Check sheet for the modelled part. Datum: model origin and axes. Units: mm. Face numbers are marked on the shaded views. A direction names the side the tool comes from. Round coordinates to 2 decimals unless told otherwise and drop trailing zeros. Order: outer loops, then holes, each group sorted by start corner. A loop starts at its lowest first (then second) coordinate and runs counter-clockwise, first axis right, second up. Notation, with made-up numbers: (36, -17.75) -> (50, -17.75) arc R10 cw to (50, -3.75) -> close; hole circle Ø10 at (11, -6.75). An arc over 180 degrees is marked (long way). Answer in a Markdown table with one row per item.
from build123d import *
from build123d.topology import SkipClean

# Parameters (mm, degrees)
SKETCH1_R           = 2
SKETCH1_R_2         = 2.5
BOSS_EXTRUDE1_DEPTH = 5
SKETCH2_R           = 3
CUT_EXTRUDE2_DEPTH  = 5
SKETCH6_R           = 40
SKETCH6_R_2         = 38
BOSS_EXTRUDE2_DEPTH = 10
CUT_EXTRUDE3_DEPTH  = 29
FILLET1_R           = 5


with BuildPart() as part:
    # Sketch1 → Boss-Extrude1 (new, symmetric)
    with SkipClean():  # the faces are left unmerged after this step: merging them gives an invalid solid
        with BuildSketch(Plane.XY):
            with BuildLine():
                Line((0, 40), (130, 40))
                ThreePointArc((130, 40), (170, 0), (130, -40))
                Line((130, -40), (0, -40))
                ThreePointArc((0, -40), (-40, 0), (0, 40))
            make_face()
            with Locations((0, 34)):
                Circle(SKETCH1_R, mode=Mode.SUBTRACT)
            with Locations((29.444863729, 17)):
                Circle(SKETCH1_R, mode=Mode.SUBTRACT)
            with Locations((29.444863729, -17)):
                Circle(SKETCH1_R, mode=Mode.SUBTRACT)
            with Locations((0, -34)):
                Circle(SKETCH1_R, mode=Mode.SUBTRACT)
            with Locations((-29.444863729, -17)):
                Circle(SKETCH1_R, mode=Mode.SUBTRACT)
            with Locations((-29.444863729, 17)):
                Circle(SKETCH1_R, mode=Mode.SUBTRACT)
            with Locations(Location((130, -34, 0), (0, 0, 180))):
                Circle(SKETCH1_R, mode=Mode.SUBTRACT)
            with Locations(Location((159.444863729, 17, 0), (0, 0, 180))):
                Circle(SKETCH1_R, mode=Mode.SUBTRACT)
            with Locations(Location((159.444863729, -17, 0), (0, 0, 180))):
                Circle(SKETCH1_R, mode=Mode.SUBTRACT)
            with Locations(Location((100.555136271, -17, 0), (0, 0, 180))):
                Circle(SKETCH1_R, mode=Mode.SUBTRACT)
            with Locations(Location((100.555136271, 17, 0), (0, 0, 180))):
                Circle(SKETCH1_R, mode=Mode.SUBTRACT)
            with Locations(Location((130, 34, 0), (0, 0, 180))):
                Circle(SKETCH1_R, mode=Mode.SUBTRACT)
            with Locations((55, 30)):
                Circle(SKETCH1_R_2, mode=Mode.SUBTRACT)
            with Locations(Location((75, 30, 0), (0, 0, 180))):
                Circle(SKETCH1_R_2, mode=Mode.SUBTRACT)
            with Locations((75, -30)):
                Circle(SKETCH1_R_2, mode=Mode.SUBTRACT)
            with Locations(Location((55, -30, 0), (0, 0, 180))):
                Circle(SKETCH1_R_2, mode=Mode.SUBTRACT)
            with BuildLine():
                ThreePointArc((25, 0), (0, 25), (-25, 0))
                ThreePointArc((-25, 0), (0, -25), (25, 0))
            make_face(mode=Mode.SUBTRACT)
            with BuildLine():
                ThreePointArc((155, 0), (130, -25), (105, 0))
                ThreePointArc((105, 0), (130, 25), (155, 0))
            make_face(mode=Mode.SUBTRACT)
        extrude(amount=BOSS_EXTRUDE1_DEPTH, both=True)
    add(part.part.scale(1), mode=Mode.REPLACE)  # the faces are merged on a copy

    # Sketch2 → Cut-Extrude2 (cut)
    with BuildSketch(Plane(origin=(0, 0, -5), x_dir=(-1, 0, 0), z_dir=(0, 0, -1))):
        with Locations((-130, 34)):
            Circle(SKETCH2_R)
        with Locations((-100.555136271, 17)):
            Circle(SKETCH2_R)
        with Locations((-100.555136271, -17)):
            Circle(SKETCH2_R)
        with Locations((-130, -34)):
            Circle(SKETCH2_R)
        with Locations((-159.444863729, -17)):
            Circle(SKETCH2_R)
        with Locations((-159.444863729, 17)):
            Circle(SKETCH2_R)
        with Locations(Location((29.444863729, 17, 0), (0, 0, 180))):
            Circle(SKETCH2_R)
        with Locations(Location((29.444863729, -17, 0), (0, 0, 180))):
            Circle(SKETCH2_R)
        with Locations(Location((0, -34, 0), (0, 0, 180))):
            Circle(SKETCH2_R)
        with Locations(Location((-29.444863729, -17, 0), (0, 0, 180))):
            Circle(SKETCH2_R)
        with Locations(Location((-29.444863729, 17, 0), (0, 0, 180))):
            Circle(SKETCH2_R)
        with Locations(Location((0, 34, 0), (0, 0, 180))):
            Circle(SKETCH2_R)
    extrude(amount=-CUT_EXTRUDE2_DEPTH, mode=Mode.SUBTRACT)

    # Sketch6 → Boss-Extrude2 (add)
    # profile 1 of 2: a face of its own
    with SkipClean():  # the faces are left unmerged after this step: merging them gives an invalid solid
        with BuildSketch(Plane.XY.offset(-5)):
            with Locations(Location((0, 0, 0), (0, 0, 90))):
                Circle(SKETCH6_R)
            Circle(SKETCH6_R_2, mode=Mode.SUBTRACT)
        # profile 2 of 2: a face of its own
        with BuildSketch(Plane.XY.offset(-5)):
            with Locations(Location((130, 0, 0), (0, 0, 180))):
                Circle(SKETCH6_R)
            with Locations((130, 0)):
                Circle(SKETCH6_R_2, mode=Mode.SUBTRACT)
        extrude(amount=-BOSS_EXTRUDE2_DEPTH)
    add(part.part.scale(1), mode=Mode.REPLACE)  # the faces are merged on a copy

    # Sketch7 → Cut-Extrude3 (cut)
    with SkipClean():  # the faces are left unmerged after this step: merging them gives an invalid solid
        with BuildSketch(Plane.XY.offset(5)):
            with BuildLine():
                Line((0, 52.799950915), (130, 52.799950915))
                Line((130, 52.799950915), (130, 40))
                ThreePointArc((130, 40), (101.715728753, 28.284271247), (90, 0))
                Line((90, 0), (90, -8.75))
                Line((90, -8.75), (40, -8.75))
                Line((40, -8.75), (40, 0))
                ThreePointArc((40, 0), (28.284271247, 28.284271247), (0, 40))
                Line((0, 40), (0, 52.799950915))
            make_face()
        extrude(amount=-CUT_EXTRUDE3_DEPTH, mode=Mode.SUBTRACT)

    # Fillet1
    fillet1_edges = [part.edges().sort_by_distance(p)[0] for p in [
        (90, -8.75, 0),
        (40, -8.75, 0),
    ]]
    fillet(fillet1_edges, radius=FILLET1_R)


solid = part.part
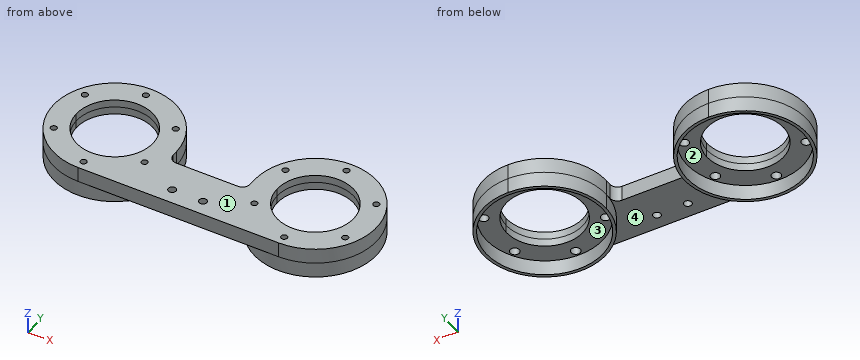
Item 1: Scan lines: line 1 (X direction, y = 36.5, z = -3.75); line 2 (X direction, y = -12, z = -8.5); line 3 (X direction, y = -35, z = -3.75). Record each from-to range of solid material in increasing order. Write a range as [from, to].
Result sheet:
| item | result |
|---|---|
| line 1 | x = [-16.36, -1.66], [1.66, 16.36], [113.64, 128.34], [131.66, 146.36] |
| line 2 | x = [-38.16, -36.06], [36.06, 38.16], [91.84, 93.94], [166.06, 168.16] |
| line 3 | x = [-19.36, -2.83], [2.83, 127.17], [132.83, 149.36] |
Item 2: Cross-section at D-D (y = -23). Record the boundary of the cut face in (x, z).
Result sheet:
| item | result |
|---|---|
| outline | (-32.73, -15) -> (-30.25, -15) -> (-30.25, -5) -> (-9.8, -5) -> (-9.8, 5) -> (-32.73, 5) -> close; (9.8, -5) -> (30.25, -5) -> (30.25, -15) -> (32.73, -15) -> (32.73, -5) -> (97.27, -5) -> (97.27, -15) -> (99.75, -15) -> (99.75, -5) -> (120.2, -5) -> (120.2, 5) -> (9.8, 5) -> close; (139.8, -5) -> (160.25, -5) -> (160.25, -15) -> (162.73, -15) -> (162.73, 5) -> (139.8, 5) -> close |
Item 3: Cross-section at C-C (z = -2.75). State how many separate pieces and enclosed holes the cut face has, and give its area (3 significant figures).
Result sheet:
| item | result |
|---|---|
| separate pieces | 1 |
| enclosed holes | 16 |
| area | 8,010 mm^2 |
Item 4: Cross-section at A-A (x = 55). Record the boundary of the cut face in (y, z), and give its area (4 significant figures).
Result sheet:
| item | result |
|---|---|
| outline | (-40, -5) -> (-32.5, -5) -> (-32.5, 5) -> (-40, 5) -> close; (-27.5, -5) -> (-8.75, -5) -> (-8.75, 5) -> (-27.5, 5) -> close |
| area | 262.5 mm^2 |
Item 5: Set-up check for the marked faces 3 and 4: record each of +Z, -Z, +X, -X, +Y, -Y from which the full face is reachable in a straight line by a thin tool's end or side.
Result sheet:
| item | result |
|---|---|
| face 3 | -Z |
| face 4 | -Z, -Y |
Item 6: Mould release check, pull along X, two halves, no side actions. Record for the marked faces 1 and 2: pulls with the +X half, pulls with the -X half, needs draft (parallel to the pull), parting line crosses it, or undercut.
Result sheet:
| item | result |
|---|---|
| face 1 | needs draft |
| face 2 | undercut |
Item 7: Cross-section at B-B (y = 4). Record the boundary of the cut face in (x, z), and give its area (3 significant figures).
Result sheet:
| item | result |
|---|---|
| outline | (-39.8, -15) -> (-37.79, -15) -> (-37.79, -5) -> (-24.68, -5) -> (-24.68, 5) -> (-39.8, 5) -> close; (24.68, -5) -> (37.79, -5) -> (37.79, -15) -> (39.8, -15) -> (39.8, 5) -> (24.68, 5) -> close; (90.2, -15) -> (92.21, -15) -> (92.21, -5) -> (105.32, -5) -> (105.32, 5) -> (90.2, 5) -> close; (154.68, -5) -> (167.79, -5) -> (167.79, -15) -> (169.8, -15) -> (169.8, 5) -> (154.68, 5) -> close |
| area | 685 mm^2 |
Item 8: Depth check by flat-ended pin: P1, Ø2.5, axis at x = 130, y = 34, coming from the -Z side; P2, Ø3, axis at x = 42, z = -1.5, coming from the +Y side; P3, Ø4.5, axis at x = 29.44, y = -17, coming from the +Z side; P4, Ø1.8, axis at x = 131.5, y = -33, coming from the -Z side. Enter the tip coordinate at first touch or a pass-through.
Result sheet:
| item | result |
|---|---|
| P1 | passes through |
| P2 | stops at y = -5.93 |
| P3 | stops at z = 5 |
| P4 | stops at z = 0 |
